Geometry check sheet. Reference: the model listing, model coordinates, mm. A direction names the side the tool comes from. Give positions to 0.01 mm unless a question says otherwise; leave off trailing zeros. Loops run counter-clockwise (first coordinate to the right, second up) from the corner with the lowest first, then second, coordinate; pieces in that order, holes last. Notation, with made-up numbers: (-38.75, -1.5) -> (-32.75, -1.5) arc R33 ccw to (-32.75, 30.5) -> close; hole circle Ø6 at (78, 17). An arc over 180 degrees is marked (long way). One line per question, with ' | ' between items.
from build123d import *

# Parameters (mm, degrees)
SKETCH_W        = 113
SKETCH_H        = 28
SKETCH_R        = 1.6
PAD_DEPTH       = 10
SKETCH001_W     = 93.6
SKETCH001_H     = 28
SKETCH001_W_2   = 5.2
SKETCH001_H_2   = 5.2
PAD001_DEPTH    = 2
POCKET_DEPTH    = 113.001
SKETCH003_W     = 5.2
SKETCH003_H     = 7.2
POCKET001_DEPTH = 1
POCKET002_DEPTH = 28.001


with BuildPart() as part:
    # Sketch → Pad (new body)
    with BuildSketch(Plane.XY):
        with Locations((41.5, 7)):
            Rectangle(SKETCH_W, SKETCH_H)
        Circle(SKETCH_R, mode=Mode.SUBTRACT)
        with Locations((0, 14)):
            Circle(SKETCH_R, mode=Mode.SUBTRACT)
        with Locations((16.6, 0)):
            Circle(SKETCH_R, mode=Mode.SUBTRACT)
        with Locations((16.6, 14)):
            Circle(SKETCH_R, mode=Mode.SUBTRACT)
        with Locations((33.2, 0)):
            Circle(SKETCH_R, mode=Mode.SUBTRACT)
        with Locations((33.2, 14)):
            Circle(SKETCH_R, mode=Mode.SUBTRACT)
        with Locations((49.8, 0)):
            Circle(SKETCH_R, mode=Mode.SUBTRACT)
        with Locations((49.8, 14)):
            Circle(SKETCH_R, mode=Mode.SUBTRACT)
        with Locations((66.4, 0)):
            Circle(SKETCH_R, mode=Mode.SUBTRACT)
        with Locations((66.4, 14)):
            Circle(SKETCH_R, mode=Mode.SUBTRACT)
        with Locations((83, 0)):
            Circle(SKETCH_R, mode=Mode.SUBTRACT)
        with Locations((83, 14)):
            Circle(SKETCH_R, mode=Mode.SUBTRACT)
    extrude(amount=PAD_DEPTH)

    # Sketch001 → Pad001 (join)
    with BuildSketch(Plane.XY):
        with Locations((41.5, 7)):
            Rectangle(SKETCH001_W, SKETCH001_H)
        Rectangle(SKETCH001_W_2, SKETCH001_H_2, mode=Mode.SUBTRACT)
        with Locations((0, 14)):
            Rectangle(SKETCH001_W_2, SKETCH001_H_2, mode=Mode.SUBTRACT)
        with Locations((16.6, 0)):
            Rectangle(SKETCH001_W_2, SKETCH001_H_2, mode=Mode.SUBTRACT)
        with Locations((16.6, 14)):
            Rectangle(SKETCH001_W_2, SKETCH001_H_2, mode=Mode.SUBTRACT)
        with Locations((33.2, 0)):
            Rectangle(SKETCH001_W_2, SKETCH001_H_2, mode=Mode.SUBTRACT)
        with Locations((33.2, 14)):
            Rectangle(SKETCH001_W_2, SKETCH001_H_2, mode=Mode.SUBTRACT)
        with Locations((49.8, 0)):
            Rectangle(SKETCH001_W_2, SKETCH001_H_2, mode=Mode.SUBTRACT)
        with Locations((49.8, 14)):
            Rectangle(SKETCH001_W_2, SKETCH001_H_2, mode=Mode.SUBTRACT)
        with Locations((66.4, 0)):
            Rectangle(SKETCH001_W_2, SKETCH001_H_2, mode=Mode.SUBTRACT)
        with Locations((66.4, 14)):
            Rectangle(SKETCH001_W_2, SKETCH001_H_2, mode=Mode.SUBTRACT)
        with Locations((83, 0)):
            Rectangle(SKETCH001_W_2, SKETCH001_H_2, mode=Mode.SUBTRACT)
        with Locations((83, 14)):
            Rectangle(SKETCH001_W_2, SKETCH001_H_2, mode=Mode.SUBTRACT)
    extrude(amount=-PAD001_DEPTH)

    # Sketch002 (on Face2 of Pad001) → Pocket (cut, through all)
    with BuildSketch(Plane(origin=(-15, 0, 0), x_dir=(0, -1, 0), z_dir=(-1, 0, 0))):
        Polygon((-21, 8), (-21, 2), (-18, 5), align=None)
        Polygon((7, 2), (7, 8), (4, 5), align=None)
    extrude(amount=-POCKET_DEPTH, mode=Mode.SUBTRACT)

    # Sketch003 → Pocket001 (cut)
    with BuildSketch(Plane.XY.offset(-2)):
        Rectangle(SKETCH003_W, SKETCH003_H)
        with Locations((0, 14)):
            Rectangle(SKETCH003_W, SKETCH003_H)
        with Locations((16.6, 0)):
            Rectangle(SKETCH003_W, SKETCH003_H)
        with Locations((16.6, 14)):
            Rectangle(SKETCH003_W, SKETCH003_H)
        with Locations((33.2, 0)):
            Rectangle(SKETCH003_W, SKETCH003_H)
        with Locations((33.2, 14)):
            Rectangle(SKETCH003_W, SKETCH003_H)
        with Locations((49.8, 0)):
            Rectangle(SKETCH003_W, SKETCH003_H)
        with Locations((49.8, 14)):
            Rectangle(SKETCH003_W, SKETCH003_H)
        with Locations((66.4, 0)):
            Rectangle(SKETCH003_W, SKETCH003_H)
        with Locations((66.4, 14)):
            Rectangle(SKETCH003_W, SKETCH003_H)
        with Locations((83, 0)):
            Rectangle(SKETCH003_W, SKETCH003_H)
        with Locations((83, 14)):
            Rectangle(SKETCH003_W, SKETCH003_H)
    extrude(amount=POCKET001_DEPTH, mode=Mode.SUBTRACT)

    # Sketch004 (on Face16 of Pocket001) → Pocket002 (cut, through all)
    with BuildSketch(Plane.XZ.offset(7)):
        Polygon((98, 8), (95, 5), (98, 2), align=None)
        Polygon((-15, 8), (-12, 5), (-15, 2), align=None)
    extrude(amount=-POCKET002_DEPTH, mode=Mode.SUBTRACT)


solid = part.part
Item 1: Sectioned sample at A-A (x = 0). Give the number of separate pieces and of enclosed holes in the cut face, plus the area to 3 significant figures.
Result:
separate pieces: 3 | enclosed holes: 0 | area: 229 mm2
Item 2: Scan lines: probe 1 along Y at (x, z) = (83, 7.75); probe 2 along Z at (x, y) = (-6, 4.25); probe 3 along X at (y, z) = (5, -0.75). Record each from-to range of solid material in increasing order.
Result:
probe 1: -6.75 to -1.6, 1.6 to 12.4, 15.6 to 20.75 | probe 2: 0 to 10 | probe 3: -5.3 to 88.3
Item 3: Set-up check for faces 4 (the face through (93, 7, 0)), 5 (the face through (-2.6, 14, -1)), 6 (the face through (96, 7, 4)), 7 (the face through (84.526, 14.481, 4.93)), 8 (the face through (41, -6, 7)): record each of +Z, -Z, +X, -X, +Y, -Y from which the full face is reachable in a straight line by a thin tool's end or side.
Result:
face 4: -Z, +X, +Y, -Y | face 5: -Z | face 6: +X, +Y, -Y | face 7: +Z, -Z | face 8: +X, -X, -Y
Item 4: Sectioned sample at C-C (x = 71.5). Record the cut outline in (y, z), plus the area to 3 significant figures.
Result:
outline: (-7, -2) -> (21, -2) -> (21, 2) -> (18, 5) -> (21, 8) -> (21, 10) -> (-7, 10) -> (-7, 8) -> (-4, 5) -> (-7, 2) -> close | area: 318 mm2
Item 5: Release check for a two-part mould opening along Z. For faces 1 (the face through (81, 0, 0)), 2 (the face through (2.6, 0, -1)), 3 (the face through (41, -5, 4)) record: pulls with the +Z half, pulls with the -Z half, needs draft (parallel to the pull), parting line crosses it, or undercut.
Result:
face 1: pulls with the -Z half | face 2: needs draft | face 3: undercut
Item 6: Depth check by flat-ended pin: pin 1 Ø1.1 at (x, y) = (84, 3) entering from -Z; pin 2 Ø2.5 at (x, y) = (-0.5, 1) entering from -Z. Enter the tip coordinate at first touch or a pass-through.
Result:
pin 1: z = -1 | pin 2: z = 0
